from build123d import *

# Parameters (mm, degrees)
CROQUIS5_W              = 660.4
CROQUIS5_H              = 25.4
SALIENTE_EXTRUIR1_DEPTH = 25.4
CROQUIS6_W              = 50.8
CROQUIS6_H              = 133.35
SALIENTE_EXTRUIR2_DEPTH = 25.4
VACIADO1_T              = -3.175
VACIADO2_T              = -3.175
CROQUIS7_R              = 2.4892
CORTAR_EXTRUIR1_DEPTH   = 402.404309499
CROQUIS9_W              = 489.4072
CROQUIS9_H              = 50.8
SALIENTE_EXTRUIR3_DEPTH = 25.4
VACIADO3_T              = -1.5875
CROQUIS10_R             = 2.4892
CROQUIS10_R_2           = 14.3129
CORTAR_EXTRUIR2_DEPTH   = 25.4
CROQUIS11_R             = 2.5527
CORTAR_EXTRUIR3_DEPTH   = 463.075777967
CROQUIS49_R             = 2.4892
CORTAR_EXTRUIR19_DEPTH  = 463.075777967
MATRIZC1_COUNT          = 2
MATRIZC1_ANGLE          = 90
CROQUIS50_R             = 2.38125
CORTAR_EXTRUIR20_DEPTH  = 463.075777967


with BuildPart() as part:
    # Croquis5 → Saliente-Extruir1 (new body)
    with BuildSketch(Plane.XY):
        with Locations((0, 80.772)):
            Rectangle(CROQUIS5_W, CROQUIS5_H)
    extrude(amount=-SALIENTE_EXTRUIR1_DEPTH)

    # Vaciado2
    vaciado2_openings = [part.faces().sort_by_distance(p)[0] for p in [
        (330.2, 80.772, -12.7),
        (-330.2, 80.772, -12.7),
    ]]
    offset(amount=VACIADO2_T, openings=vaciado2_openings, kind=Kind.INTERSECTION)


with BuildPart() as body_2:
    # Croquis6 → Saliente-Extruir2 (new body)
    with BuildSketch(Plane.XY):
        with Locations((0, 160.147)):
            Rectangle(CROQUIS6_W, CROQUIS6_H)
    extrude(amount=-SALIENTE_EXTRUIR2_DEPTH)

    # Vaciado1
    vaciado1_openings = [body_2.faces().sort_by_distance(p)[0] for p in [
        (0, 226.822, -12.7),
        (0, 93.472, -12.7),
    ]]
    offset(amount=VACIADO1_T, openings=vaciado1_openings, kind=Kind.INTERSECTION)

    # Croquis7 → Cortar-Extruir1 (cut, through all)
    with BuildSketch(Plane.XY):
        with Locations((0, 199.8345)):
            Circle(CROQUIS7_R)
        with Locations((0, 152.2095)):
            Circle(CROQUIS7_R)
        with BuildLine():
            Line((-11.1506, 158.5214), (11.1506, 158.5214))
            ThreePointArc((11.1506, 158.5214), (15.640728061, 160.381271939), (17.5006, 164.8714))
            Line((17.5006, 164.8714), (17.5006, 187.1726))
            ThreePointArc((17.5006, 187.1726), (15.640728061, 191.662728061), (11.1506, 193.5226))
            Line((11.1506, 193.5226), (-11.1506, 193.5226))
            ThreePointArc((-11.1506, 193.5226), (-15.640728061, 191.662728061), (-17.5006, 187.1726))
            Line((-17.5006, 187.1726), (-17.5006, 164.8714))
            ThreePointArc((-17.5006, 164.8714), (-15.640728061, 160.381271939), (-11.1506, 158.5214))
        make_face()
    extrude(amount=-CORTAR_EXTRUIR1_DEPTH, mode=Mode.SUBTRACT)


with BuildPart() as body_3:
    # Croquis9 → Saliente-Extruir3 (new, symmetric)
    with BuildSketch(Plane(origin=(0, 0, -85.440650048), x_dir=(-1, 0, 0), z_dir=(0, 0, -1))):
        with Locations((168.0464, 176.022)):
            Rectangle(CROQUIS9_W, CROQUIS9_H)
    extrude(amount=SALIENTE_EXTRUIR3_DEPTH, both=True)

    # Vaciado3
    vaciado3_openings = [body_3.faces().sort_by_distance(p)[0] for p in [
        (-412.75, 176.022, -85.440650048),
        (76.6572, 176.022, -85.440650048),
    ]]
    offset(amount=VACIADO3_T, openings=vaciado3_openings, kind=Kind.INTERSECTION)

    # Croquis10 → Cortar-Extruir2 (cut, symmetric)
    with BuildSketch(Plane.XY.offset(-85.440650048)):
        with Locations(Location((-20.622229928, 187.92825, 0), (0, 0, 180))):
            Circle(CROQUIS10_R)
        with Locations(Location((-20.622229928, 164.11575, 0), (0, 0, 180))):
            Circle(CROQUIS10_R)
        with Locations((20.622229928, 164.11575)):
            Circle(CROQUIS10_R)
        with Locations(Location((20.622229928, 187.92825, 0), (0, 0, 180))):
            Circle(CROQUIS10_R)
        with Locations(Location((0, 176.022, 0), (0, 0, 180))):
            Circle(CROQUIS10_R_2)
    extrude(amount=CORTAR_EXTRUIR2_DEPTH, both=True, mode=Mode.SUBTRACT)

    # Croquis11 → Cortar-Extruir3 (cut, through all)
    with BuildSketch(Plane.XY.offset(-60.040650048)):
        with Locations((-50.8, 188.722)):
            Circle(CROQUIS11_R)
        with Locations((-50.8, 176.022)):
            Circle(CROQUIS11_R)
        with Locations((-50.8, 163.322)):
            Circle(CROQUIS11_R)
        with Locations((50.8, 163.322)):
            Circle(CROQUIS11_R)
        with Locations((50.8, 176.022)):
            Circle(CROQUIS11_R)
        with Locations((50.8, 188.722)):
            Circle(CROQUIS11_R)
    extrude(amount=-CORTAR_EXTRUIR3_DEPTH, mode=Mode.SUBTRACT)

    # Croquis49 → Cortar-Extruir19 (cut, through all)
    with BuildSketch(Plane(origin=(0, 0, -110.840650048), x_dir=(-1, 0, 0), z_dir=(0, 0, -1))):
        with Locations((407.9875, 195.072)):
            Circle(CROQUIS49_R)
        with Locations((407.9875, 176.022)):
            Circle(CROQUIS49_R)
        with Locations((407.9875, 156.972)):
            Circle(CROQUIS49_R)
        with Locations((395.2875, 195.072)):
            Circle(CROQUIS49_R)
        with Locations((395.2875, 176.022)):
            Circle(CROQUIS49_R)
        with Locations((395.2875, 156.972)):
            Circle(CROQUIS49_R)
        with Locations((382.5875, 195.072)):
            Circle(CROQUIS49_R)
        with Locations((382.5875, 176.022)):
            Circle(CROQUIS49_R)
        with Locations((382.5875, 156.972)):
            Circle(CROQUIS49_R)
    cortar_extruir19 = extrude(amount=-CORTAR_EXTRUIR19_DEPTH, mode=Mode.SUBTRACT)

    # MatrizC1: Cortar-Extruir19 ×2 about axis
    matrizc1_axis = Axis((101.12756, 176.022, -85.440650048), (-1, 0, 0))
    for i in range(1, MATRIZC1_COUNT):
        add(cortar_extruir19.rotate(matrizc1_axis, i * MATRIZC1_ANGLE / (MATRIZC1_COUNT - 1)), mode=Mode.SUBTRACT)

    # Croquis50 → Cortar-Extruir20 (cut, through all)
    with BuildSketch(Plane(origin=(0, 0, -110.840650048), x_dir=(-1, 0, 0), z_dir=(0, 0, -1))):
        with Locations((326.91705, 167.29075)):
            Circle(CROQUIS50_R)
        with Locations((326.91705, 184.75325)):
            Circle(CROQUIS50_R)
        with Locations((257.68935, 167.29075)):
            Circle(CROQUIS50_R)
        with Locations((257.68935, 184.75325)):
            Circle(CROQUIS50_R)
        with Locations((188.46165, 167.29075)):
            Circle(CROQUIS50_R)
        with Locations((188.46165, 184.75325)):
            Circle(CROQUIS50_R)
        with Locations((119.23395, 167.29075)):
            Circle(CROQUIS50_R)
        with Locations((119.23395, 184.75325)):
            Circle(CROQUIS50_R)
    extrude(amount=-CORTAR_EXTRUIR20_DEPTH, mode=Mode.SUBTRACT)


solid = body_3.part
Source: CAD feature listing. Evaluate the final solid. Frame: model axes, mm. A direction names the side the tool comes from. Round coordinates to 2 decimals unless told otherwise and drop trailing zeros. Loops run counter-clockwise (first coordinate to the right, second up) from the corner with the lowest first, then second, coordinate; pieces in that order, holes last.
Q1. Ray query, line 1 (Y direction, x = 50.8, z = -109.55); line 2 (Z direction, x = -76, y = 173); line 3 (Y direction, x = -264.5, z = -73.5). Return the intervals inside material, ascending.
Q2. Section A-A, the plane z = -77. Return loops of the section in (x, y), plus the area to 3 significant figures.
Q3. First-contact query: P1, Ø1, axis at x = 12, y = 182, coming from the +Z side. Flat tip, straight axial feed; report the tip coordinate or a pass-through.
Q4. Mould query, pull axis Y, two halves, no side actions, for faces 3 (the face through (-165, 150.622, -86)), 4 (the face through (-165, 201.422, -86)), 5 (the face through (-165, 176, -110.841)), 6 (the face through (1.86, 161.83, -110.04)). Classes: pulls with the +Y half, pulls with the -Y half, needs draft (parallel to the pull), parting line crosses it, or undercut.
Q5. Section B-B, the plane x = 0. Return loops of the section in (y, z), plus the area to 3 significant figures.
Q6. Access query for faces 1 (the face through (-165, 199.834, -86)), 2 (the face through (76.657, 174, -61)). Directions: +Z, -Z, +X, -X, +Y, -Y. A direction counts if a zero-diameter tool reaches every point of the face in a straight line with its end or side. Return the directions, or none.
Solutions:
1. line 1: y = 150.62 to 160.77, 165.87 to 173.47, 178.57 to 186.17, 191.27 to 201.42
1. line 2: z = -110.84 to -109.25, -61.63 to -60.04
1. line 3: y = 150.62 to 152.21, 199.83 to 201.42
2. outline: (-412.75, 150.62) - (76.66, 150.62) - (76.66, 152.21) - (-412.75, 152.21) - close; (-412.75, 199.83) - (76.66, 199.83) - (76.66, 201.42) - (-412.75, 201.42) - close
2. area: 1,550 mm2
3. P1: passes through
4. face 3: pulls with the -Y half
4. face 4: pulls with the +Y half
4. face 5: needs draft
4. face 6: undercut
5. outline: (150.62, -110.84) - (161.71, -110.84) - (161.71, -109.25) - (152.21, -109.25) - (152.21, -61.63) - (161.71, -61.63) - (161.71, -60.04) - (150.62, -60.04) - close; (190.33, -110.84) - (201.42, -110.84) - (201.42, -60.04) - (190.33, -60.04) - (190.33, -61.63) - (199.83, -61.63) - (199.83, -109.25) - (190.33, -109.25) - close
5. area: 222 mm2
6. face 1: +X, -X
6. face 2: +Z, -Z, +X, +Y, -Y
